```python
from build123d import *

# Parameters (mm, degrees)
SKETCH_W        = 20
SKETCH_H        = 20
SKETCH_R        = 2.6
PAD_DEPTH       = 3
SKETCH001_R     = 3.9
SKETCH001_R_2   = 2.6
PAD001_DEPTH    = 6
PAD002_DEPTH    = 20
PAD002_FACE16_R = 2.6
POCKET_DEPTH    = 6.001
FILLET_R        = 3


with BuildPart() as part:
    # Sketch → Pad (new body)
    with BuildSketch(Plane.XY):
        Rectangle(SKETCH_W, SKETCH_H)
        Circle(SKETCH_R, mode=Mode.SUBTRACT)
    extrude(amount=PAD_DEPTH)

    # Sketch001 (on Face6 of Pad) → Pad001 (join)
    with BuildSketch(Plane(origin=(0, 0, 0), x_dir=(1, 0, 0), z_dir=(0, 0, -1))):
        Circle(SKETCH001_R)
        Circle(SKETCH001_R_2, mode=Mode.SUBTRACT)
    extrude(amount=PAD001_DEPTH)

    # Sketch002 (on Face1 of Pad001) → Pad002 (join)
    with BuildSketch(Plane(origin=(0, 10, 0), x_dir=(-1, 0, 0), z_dir=(0, 1, 0))):
        Polygon((-4.75, 0), (4.75, 0), (2.95, -1.5), (-2.95, -1.5), align=None)
    extrude(amount=-PAD002_DEPTH)

    # Pad002 Face16 → Pocket (cut, through all)
    with BuildSketch(Plane(origin=(0, 0, 0), x_dir=(0, 1, 0), z_dir=(0, 0, 1))):
        Circle(PAD002_FACE16_R)
    extrude(amount=-POCKET_DEPTH, mode=Mode.SUBTRACT)

    # Fillet
    fillet_edges = [part.edges().sort_by_distance(p)[0] for p in [
        (10, -10, 1.5),
        (-10, -10, 1.5),
        (10, 10, 1.5),
        (-10, 10, 1.5),
    ]]
    fillet(fillet_edges, radius=FILLET_R)


solid = part.part
```
Read the model definition and answer for the solid it produces. Units are mm, in the model's axes. A direction names the side the tool comes from. Round coordinates to 2 decimals unless told otherwise and drop trailing zeros. Write each loop counter-clockwise with the first axis right and the second up, starting at its lowest first coordinate (ties: lowest second). Pieces come first, ordered by that corner, then holes. Notation, with made-up numbers: (80.5, 28) - (94.5, 28) arc R12 cw to (94.5, 35) - close; hole circle Ø6 at (-27.5, 61). An arc over 180 degrees is marked (long way). One line per item, written item: value.
Q1. Find section B-B (x = -3.25). Determine the outline of the cut face in (y, z), and give its area (3 significant figures).
The answers:
outline: (-10, -1.25) - (-2.16, -1.25) - (-2.16, -6) - (2.16, -6) - (2.16, -1.25) - (10, -1.25) - (10, 3) - (-10, 3) - close
area: 105 mm2
Q2. Find section C-C (y = 3.25). Determine the outline of the cut face in (x, z), and give its area (3 significant figures).
The answers:
outline: (-10, 0) - (-4.75, 0) - (-2.95, -1.5) - (-2.16, -1.5) - (-2.16, -6) - (2.16, -6) - (2.16, -1.5) - (2.95, -1.5) - (4.75, 0) - (10, 0) - (10, 3) - (-10, 3) - close
area: 91.0 mm2
Q3. Which of the six approach directions +Z, -Z, +X, -X, +Y, -Y give full straight-line access (tool end or side, diameter ignored) to faces 1 (the flat face through (-7, 0, 0)), 2 (the flat face through (7, 0, 0)), 3 (the flat face through (-4.063, 0.14, -0.573))?
The answers:
face 1: -Z, -X, +Y, -Y
face 2: -Z, +X, +Y, -Y
face 3: -Z, -X
Q4. Find section D-D (z = -5.5). Determine the outline of the cut face in (x, y).
The answers:
outline: circle Ø7.8 at (0, 0); hole circle Ø5.2 at (0, 0)
Q5. Each of these flat-tipped pins is pushed along its axis until it touches: P1, Ø1.6, axis at x = -8, y = -1.5, coming from the -Z side; P2, Ø1.5, axis at x = -1, y = 5, coming from the -Z side; P3, Ø1.5, axis at y = 0, z = -4.5, coming from the +X side. Where does it stop, or does it pass through?
The answers:
P1: stops at z = 0
P2: stops at z = -1.5
P3: stops at x = 3.9
Q6. Straight lines are drawn through the part: line 1 (X direction, y = 0, z = -4.85); line 2 (Y direction, x = 0, z = 1.15). For each, find the intervals that lie inside material, in ascending order. Write a range as from..to.
The answers:
line 1: x = -3.9..-2.6, 2.6..3.9
line 2: y = -10..-2.6, 2.6..10
Q7. Find section A-A (z = -0.25). Determine the outline of the cut face in (x, y).
The answers:
outline: (-4.45, -10) - (4.45, -10) - (4.45, 10) - (-4.45, 10) - close; hole circle Ø5.2 at (0, 0)
